Design review of the part built by this model. Coordinates are the model's own, in mm. A direction names the side the tool comes from. Coordinates: 2 decimals unless noted, no trailing zeros. Write each loop counter-clockwise with the first axis right and the second up, starting at its lowest first coordinate (ties: lowest second). Pieces come first, ordered by that corner, then holes. Notation, with made-up numbers: (83.5, 1) -> (118.5, 1) arc R10 ccw to (118.5, 12) -> close; hole circle Ø5 at (-40, 83.5). An arc over 180 degrees is marked (long way). Write item = value, one per line. Start each with the question number.
```python
from build123d import *

# Parameters (mm, degrees)
SKETCH_1_W          = 72
SKETCH_1_H          = 32.9
EXTRUDE_1_DEPTH     = 162.5
SHELL_1_T           = 1.5
FILLET_2_R          = 1
EXTRUDE_2_DEPTH     = 4.5
SKETCH_8_R          = 1.1
CUT_EXTRUDE_3_DEPTH = 5
CUT_EXTRUDE_4_DEPTH = 1.7
FILLET_3_R          = 1.25
SKETCH_11_W         = 0.5
SKETCH_11_H         = 1
CUT_EXTRUDE_5_DEPTH = 1.7
FILLET_4_R          = 0.2
FILLET_5_R          = 0.1


with BuildPart() as part:
    # 草图1 → 凸台-拉伸1 (new body)
    with BuildSketch(Plane(origin=(0, 0, 0), x_dir=(1, 0, 0), z_dir=(0, 1, 0))):
        with Locations((36, 16.45)):
            Rectangle(SKETCH_1_W, SKETCH_1_H)
    extrude(amount=EXTRUDE_1_DEPTH)

    # 抽壳1
    shell_1_openings = [part.faces().sort_by_distance(p)[0] for p in [
        (36, 162.5, -16.45),
    ]]
    offset(amount=SHELL_1_T, openings=shell_1_openings, kind=Kind.INTERSECTION)

    # 圆角2
    # the kernel refuses this fillet: 1 mm, written as the material it takes off along each edge
    with BuildSketch(Plane(origin=(72.5, -0.5, -33.4), x_dir=(0, -1, 0), z_dir=(0, 0, -1))) as fillet_2_piece_1_section:
        Polygon((0, 0), (FILLET_2_R, 0), (FILLET_2_R, -FILLET_2_R), (0, -FILLET_2_R), align=None)
    fillet_2_piece_1 = extrude(amount=FILLET_2_R, mode=Mode.PRIVATE)
    fillet_2_piece_1 = fillet_2_piece_1 - Plane(origin=(72.5, -0.5, -33.4), x_dir=(-0.7071067811865475, 0.7071067811865475, 0), z_dir=(0, 0, -1)) * Sphere(FILLET_2_R, mode=Mode.PRIVATE)
    add(fillet_2_piece_1, mode=Mode.SUBTRACT)
    with BuildSketch(Plane(origin=(-0.5, -0.5, -33.4), x_dir=(-1, 0, 0), z_dir=(0, 0, -1))) as fillet_2_piece_2_section:
        Polygon((0, 0), (FILLET_2_R, 0), (FILLET_2_R, -FILLET_2_R), (0, -FILLET_2_R), align=None)
    fillet_2_piece_2 = extrude(amount=FILLET_2_R, mode=Mode.PRIVATE)
    fillet_2_piece_2 = fillet_2_piece_2 - Plane(origin=(-0.5, -0.5, -33.4), x_dir=(0.7071067811865475, 0.7071067811865475, 0), z_dir=(0, 0, -1)) * Sphere(FILLET_2_R, mode=Mode.PRIVATE)
    add(fillet_2_piece_2, mode=Mode.SUBTRACT)
    with BuildSketch(Plane(origin=(72.5, -0.5, 0.5), x_dir=(0, 0, 1), z_dir=(0, -1, 0))) as fillet_2_piece_3_section:
        Polygon((0, 0), (FILLET_2_R, 0), (FILLET_2_R, -FILLET_2_R), (0, -FILLET_2_R), align=None)
    fillet_2_piece_3 = extrude(amount=FILLET_2_R, mode=Mode.PRIVATE)
    fillet_2_piece_3 = fillet_2_piece_3 - Plane(origin=(72.5, -0.5, 0.5), x_dir=(-0.7071067811865475, 0, -0.7071067811865475), z_dir=(0, -1, 0)) * Sphere(FILLET_2_R, mode=Mode.PRIVATE)
    add(fillet_2_piece_3, mode=Mode.SUBTRACT)
    with BuildSketch(Plane(origin=(-0.5, -0.5, 0.5), x_dir=(0, -1, 0), z_dir=(-1, 0, 0))) as fillet_2_piece_4_section:
        Polygon((0, 0), (FILLET_2_R, 0), (FILLET_2_R, FILLET_2_R), (0, FILLET_2_R), align=None)
    fillet_2_piece_4 = extrude(amount=FILLET_2_R, mode=Mode.PRIVATE)
    fillet_2_piece_4 = fillet_2_piece_4 - Plane(origin=(-0.5, -0.5, 0.5), x_dir=(0, 0.7071067811865475, -0.7071067811865475), z_dir=(-1, 0, 0)) * Sphere(FILLET_2_R, mode=Mode.PRIVATE)
    add(fillet_2_piece_4, mode=Mode.SUBTRACT)
    with BuildSketch(Plane(origin=(72.5, -1.5, -34.4), x_dir=(0, 1, 0), z_dir=(-1, 0, 0)), Plane(origin=(-0.5, -1.5, 1.5), x_dir=(0, 1, 0), z_dir=(1, 0, 0))) as fillet_2_piece_5:
        with BuildLine():
            CenterArc((FILLET_2_R, -FILLET_2_R), FILLET_2_R, 90, 90)
            Line((0, -FILLET_2_R), (0, 0))
            Line((0, 0), (FILLET_2_R, 0))
        make_face()
    extrude(amount=73, mode=Mode.SUBTRACT)
    with BuildSketch(Plane(origin=(73.5, -1.5, 0.5), x_dir=(0, 1, 0), z_dir=(0, 0, -1)), Plane(origin=(-1.5, -1.5, -33.4), x_dir=(0, 1, 0), z_dir=(0, 0, 1))) as fillet_2_piece_6:
        with BuildLine():
            CenterArc((FILLET_2_R, -FILLET_2_R), FILLET_2_R, 90, 90)
            Line((0, -FILLET_2_R), (0, 0))
            Line((0, 0), (FILLET_2_R, 0))
        make_face()
    extrude(amount=33.9, mode=Mode.SUBTRACT)
    with BuildSketch(Plane(origin=(-1.5, -0.5, -34.4), x_dir=(1, 0, 0), z_dir=(0, 1, 0)), Plane(origin=(73.5, -0.5, -34.4), x_dir=(0, 0, 1), z_dir=(0, 1, 0)), Plane(origin=(73.5, -0.5, 1.5), x_dir=(-1, 0, 0), z_dir=(0, 1, 0)), Plane(origin=(-1.5, 165, 1.5), x_dir=(1, 0, 0), z_dir=(0, -1, 0))) as fillet_2_piece_7:
        with BuildLine():
            CenterArc((FILLET_2_R, -FILLET_2_R), FILLET_2_R, 90, 90)
            Line((0, -FILLET_2_R), (0, 0))
            Line((0, 0), (FILLET_2_R, 0))
        make_face()
    extrude(amount=165.5, mode=Mode.SUBTRACT)

    # 草图2 → 凸台-拉伸2 (add)
    with BuildSketch(Plane(origin=(0, 162.5, 0), x_dir=(1, 0, 0), z_dir=(0, 1, 0))):
        Polygon((-1.5, 6), (-1.5, 26.9), (0.6, 26.9), (0.6, 32.9), (-4.1, 32.9), (-4.1, 26.9), (-4.1, 6), (-4.1, 0), (0.6, 0), (0.6, 6), align=None)
        Polygon((73.5, 26.9), (73.5, 6), (71.4, 6), (71.4, 0), (76.1, 0), (76.1, 6), (76.1, 26.9), (76.1, 32.9), (71.4, 32.9), (71.4, 26.9), align=None)
    extrude(amount=-EXTRUDE_2_DEPTH)

    # 草图8 → 切除-拉伸3 (cut)
    with BuildSketch(Plane(origin=(0, 162.5, 0), x_dir=(1, 0, 0), z_dir=(0, 1, 0))):
        with Locations(Location((-1.75, 29.9, 0), (0, 0, 270))):
            Circle(SKETCH_8_R)
        with Locations(Location((73.75, 29.9, 0), (0, 0, 256.863441213))):
            Circle(SKETCH_8_R)
        with Locations(Location((73.75, 3, 0), (0, 0, 270))):
            Circle(SKETCH_8_R)
        with Locations(Location((-1.75, 3, 0), (0, 0, 283.136558787))):
            Circle(SKETCH_8_R)
    extrude(amount=-CUT_EXTRUDE_3_DEPTH, mode=Mode.SUBTRACT)

    # 草图10 → 切除-拉伸4 (cut)
    with BuildSketch(Plane.XZ.offset(-158)):
        Polygon((-2.360902354, -27.8), (-4.325128869, -27.8), (-4.325128869, -32), (-2.477398874, -32), (-0.537564435, -32), (0.674871131, -29.9), (-0.537564435, -27.8), align=None)
        Polygon((76.325128869, -27.8), (76.325128869, -32), (74.477398874, -32), (72.537564435, -32), (71.325128869, -29.9), (72.537564435, -27.8), (74.360902354, -27.8), align=None)
        Polygon((-4.325128869, -5.1), (-4.325128869, -0.9), (-2.477398874, -0.9), (-0.537564435, -0.9), (0.674871131, -3), (-0.537564435, -5.1), (-2.360902354, -5.1), align=None)
        Polygon((74.360902354, -5.1), (76.325128869, -5.1), (76.325128869, -0.9), (74.477398874, -0.9), (72.537564435, -0.9), (71.325128869, -3), (72.537564435, -5.1), align=None)
    extrude(amount=-CUT_EXTRUDE_4_DEPTH, mode=Mode.SUBTRACT)

    # 圆角3
    fillet_3_edges = [part.edges().sort_by_distance(p)[0] for p in [
        (76.1, 160.25, -32.9),
        (76.1, 160.25, 0),
        (-4.1, 160.25, 0),
        (-4.1, 160.25, -32.9),
    ]]
    fillet(fillet_3_edges, radius=FILLET_3_R)

    # 草图11 → 切除-拉伸5 (cut)
    with BuildSketch(Plane.XZ.offset(-158)):
        with Locations((0.55, -3)):
            Rectangle(SKETCH_11_W, SKETCH_11_H)
        with Locations((71.45, -3)):
            Rectangle(SKETCH_11_W, SKETCH_11_H)
        with Locations((71.45, -29.9)):
            Rectangle(SKETCH_11_W, SKETCH_11_H)
        with Locations((0.55, -29.9)):
            Rectangle(SKETCH_11_W, SKETCH_11_H)
    extrude(amount=-CUT_EXTRUDE_5_DEPTH, mode=Mode.SUBTRACT)

    # 圆角4
    fillet_4_edges = [part.edges().sort_by_distance(p)[0] for p in [
        (72, 158, -31.984455543),
        (72, 158, -5.084455543),
        (72, 158, -0.915544457),
        (72, 158, -27.815544457),
        (0, 158, -0.915544457),
        (0, 158, -27.815544457),
        (0, 158, -31.984455543),
        (0, 158, -5.084455543),
    ]]
    fillet(fillet_4_edges, radius=FILLET_4_R)

    # 圆角5
    fillet_5_edges = [part.edges().sort_by_distance(p)[0] for p in [
        (0, 157.9, -28.731088913),
        (0, 157.9, -31.068911087),
        (0, 157.9, -4.168911087),
        (0, 157.9, -1.831088913),
        (72, 157.9, -4.168911087),
        (72, 157.9, -1.831088913),
        (72, 157.9, -28.731088913),
        (72, 157.9, -31.068911087),
    ]]
    fillet(fillet_5_edges, radius=FILLET_5_R)


solid = part.part
```
(1) Take a section at B-B, the plane x = 38. State the section outline as (y, z) points, then the cut area to 3 significant figures.
(2) Take a section at A-A, the plane y = 35.5. State the section outline as (x, z) points.
(3) For line 1 (X direction, y = 160.75, z = -29.9); line 2 (Z direction, x = 0.5, y = 52); line 3 (X direction, y = 137.5, z = -18.5), list the stretches that pass through material, from the lowest coordinate up.
(4) Mouldability with a two-part tool opening along Z and no side actions: class faces 1 (the face through (35, 80, -34.4)), 2 (the face through (35, 0, -17)), 3 (the face through (73.5, 80, -16)) as pulls with the +Z half, pulls with the -Z half, needs draft (parallel to the pull), parting line crosses it, or undercut.
(5) For faces 4 (the face through (71.4, 160, -3)), 5 (the face through (75, 159.7, -29)), 6 (the face through (0, 80, -16)), 7 (the face through (-3, 159.7, -2)), 8 (the face through (76.1, 160, -16)), list the 3-axis set-ups (+Z, -Z, +X, -X, +Y, -Y) from which the entire face can be reached by the end or side of a thin tool; tool diameter is ignored.
(6) For pin 1 Ø8 at (y, z) = (81, -27) entering from +X; pin 2 Ø1.4 at (x, y) = (73.5, 159.5) entering from -Z; pin 3 Ø2 at (x, z) = (-1.75, -29.9) entering from -Y, all flat-tipped, find the tip position at first contact; note any pin that passes through.
(7) Take a section at C-C, the plane z = -17.5. State the section outline as (x, y) points.
Report:
q1.outline = (-1.5, -33.4) arc R1 ccw to (-0.5, -34.4) -> (162.5, -34.4) -> (162.5, -32.9) -> (0, -32.9) -> (0, 0) -> (162.5, 0) -> (162.5, 1.5) -> (-0.5, 1.5) arc R1 ccw to (-1.5, 0.5) -> close
q1.area = 541 mm2
q2.outline = (-1.5, -33.4) arc R1 ccw to (-0.5, -34.4) -> (72.5, -34.4) arc R1 ccw to (73.5, -33.4) -> (73.5, 0.5) arc R1 ccw to (72.5, 1.5) -> (-0.5, 1.5) arc R1 ccw to (-1.5, 0.5) -> close; hole (0, -32.9) -> (72, -32.9) -> (72, 0) -> (0, 0) -> close
q3.line_1 = -4.1 to -2.85, -0.65 to 0.6, 71.4 to 72.65, 74.85 to 76.1
q3.line_2 = -34.4 to -32.9, 0 to 1.5
q3.line_3 = -1.5 to 0, 72 to 73.5
q4.face_1 = pulls with the -Z half
q4.face_2 = undercut
q4.face_3 = needs draft
q5.face_4 = +Y
q5.face_5 = +X
q5.face_6 = none
q5.face_7 = -X
q5.face_8 = +Z, -Z, +X, +Y, -Y
q6.pin_1 = 73.5
q6.pin_2 = -34.35
q6.pin_3 = -1.47
q7.outline = (-4.1, 158) -> (-1.5, 158) -> (-1.5, -0.5) arc R1 ccw to (-0.5, -1.5) -> (72.5, -1.5) arc R1 ccw to (73.5, -0.5) -> (73.5, 158) -> (76.1, 158) -> (76.1, 162.5) -> (72, 162.5) -> (72, 0) -> (0, 0) -> (0, 162.5) -> (-4.1, 162.5) -> close
